Check sheet for the modelled part. Datum: model origin and axes. Units: mm. A direction names the side the tool comes from. Give positions to 0.01 mm unless a question says otherwise; leave off trailing zeros. Loops run counter-clockwise (first coordinate to the right, second up) from the corner with the lowest first, then second, coordinate; pieces in that order, holes last. Notation, with made-up numbers: (15, -5) - (61, -5) arc R29 ccw to (61, 19) - close; hole circle Ø4 at (-13.75, -36). An arc over 180 degrees is marked (long way). Answer in a Markdown table with one row per item. Add a question column.
(1) Sectioned sample at A-A on y = 3. Enter the section's corners in (x, z).
(2) Set-up check for faces 4 (the face through (0.29, 18.47, 10.58)), 5 (the face through (-3.779, -20, 1)), 6 (the face through (-22.382, 0, 7)): record each of +Z, -Z, +X, -X, +Y, -Y from which the full face is reachable in a straight line by a thin tool's end or side.
(3) Sectioned sample at C-C on z = -4.5. State how many separate pieces and enclosed holes the cut face has, then the cut area to 3 significant figures.
(4) Thickness scan on L1, parallel to X at y = 0, z = 11.1; L2, parallel to X at y = -15, z = 8.25; L3, parallel to Y at x = 5, z = -6. Record the ranges inside material, lowest first.
(5) Sectioned sample at B-B on x = -1. Enter the section's corners in (y, z).
(6) Sectioned sample at D-D on y = 12.5. Enter the section's corners in (x, z), then the cut area to 3 significant figures.
(7) Draft check along Z on faces 1 (the face through (-21.524, 0.071, 5.623)), 2 (the face through (18.721, -20, 1)), 3 (the face through (-4.344, -18.523, -2.422)). Enter one of: released by +Z, released by -Z, zero draft, split by the parting line, or undercut.
(8) Go/stop test with flat-tipped pins: P1, Ø0.5, axis at x = -8.5, y = -20.5, coming from the -Z side; P2, Ø3, axis at x = -15.5, y = -9, coming from the +Z side; P3, Ø12, axis at x = -13.5, z = 5, coming from the -Y side; P4, Ø3, axis at x = -11.5, z = -3.5, coming from the +Y side. Record where each tip stops, or that it passes through.
from build123d import *

# Parameters (mm, degrees)
PAD_DEPTH            = 20.6929
PAD001_DEPTH         = 1.692
PAD002_DEPTH         = 1.692
PAD003_START         = -1
SKETCH003_W          = 14.9418
SKETCH003_H          = 1.0711
PAD003_DEPTH         = 20.08
PAD004_DEPTH         = 1.1445
PAD005_DEPTH         = 1.1445
PAD006_DEPTH         = 1.1445
PAD007_DEPTH         = 1.1445
SKETCH008_R          = 18
SKETCH008_R_2        = 1.625
POCKET_DEPTH         = 21.0957
POCKET_DEPTH_BACK    = 0.4219
CHAMFER001_SIZE      = 0.7
SKETCH013_R          = 1.625
POCKET001_DEPTH      = 22.383
POCKET001_DEPTH_BACK = 22.383
BODY_PLACEMENT_ANGLE = 90


with BuildPart() as part:
    # Sketch → Pad (new body, symmetric)
    with BuildSketch(Plane.YZ):
        with BuildLine():
            ThreePointArc((0, 20.5122), (-0.4209, 0), (0, -20.5122))
            ThreePointArc((0, -20.5122), (0.44097, -21.514212), (1.445369, -21.949718))
            Line((1.445369, -21.949718), (11.0791, -22.292695))
            Line((11.0791, -22.292695), (11.0791, -20.791745))
            Line((1.498737, -20.450667), (11.0791, -20.791745))
            ThreePointArc((1.498737, 20.450667), (1.0791, 0), (1.498737, -20.450667))
            Line((1.498737, 20.450667), (11.0791, 20.791745))
            Line((11.0791, 20.791745), (11.0791, 22.292695))
            Line((1.445369, 21.949718), (11.0791, 22.292695))
            ThreePointArc((1.445369, 21.949718), (0.44097, 21.514212), (0, 20.5122))
        make_face()
    extrude(amount=PAD_DEPTH, both=True)

    # Sketch001 → Pad001 (join)
    with BuildSketch(Plane.YZ.offset(20.69)):
        with BuildLine():
            ThreePointArc((0, 20.5122), (-0.4209, 0), (0, -20.5122))
            ThreePointArc((0, -20.5122), (0.44097, -21.514212), (1.445369, -21.949718))
            Line((1.445369, -21.949718), (11.0791, -22.292695))
            Line((11.0791, 22.292695), (11.0791, -22.292695))
            Line((1.445369, 21.949718), (11.0791, 22.292695))
            ThreePointArc((1.445369, 21.949718), (0.44097, 21.514212), (0, 20.5122))
        make_face()
    extrude(amount=PAD001_DEPTH)

    # Sketch002 → Pad002 (join)
    with BuildSketch(Plane.YZ.offset(-20.69)):
        with BuildLine():
            ThreePointArc((0, 20.5122), (-0.4209, 0), (0, -20.5122))
            ThreePointArc((0, -20.5122), (0.44097, -21.514212), (1.445369, -21.949718))
            Line((1.445369, -21.949718), (11.0791, -22.292695))
            Line((11.0791, 22.292695), (11.0791, -22.292695))
            Line((1.445369, 21.949718), (11.0791, 22.292695))
            ThreePointArc((1.445369, 21.949718), (0.44097, 21.514212), (0, 20.5122))
        make_face()
    extrude(amount=-PAD002_DEPTH)

    # Sketch003 → Pad003 (join)
    with BuildSketch(Plane.XZ.offset(PAD003_START)):
        with Locations((-11.25, 20.36445)):
            Rectangle(SKETCH003_W, SKETCH003_H)
        with Locations((11.25, 20.36445)):
            Rectangle(SKETCH003_W, SKETCH003_H)
        with Locations((-11.25, -20.36445)):
            Rectangle(SKETCH003_W, SKETCH003_H)
        with Locations((11.25, -20.36445)):
            Rectangle(SKETCH003_W, SKETCH003_H)
    extrude(amount=-PAD003_DEPTH)

    # Sketch004 → Pad004 (join)
    with BuildSketch(Plane.YZ.offset(3.78)):
        Polygon((1.358658, 16.220017), (1.488, 19.8289), (21.0947, 19.8289), (21.0947, 19.7), align=None)
        Polygon((1.358658, -16.220017), (1.488, -19.8289), (21.0947, -19.8289), (21.0947, -19.7), align=None)
    extrude(amount=PAD004_DEPTH)

    # Sketch005 → Pad005 (join)
    with BuildSketch(Plane.YZ.offset(-3.78)):
        Polygon((1.358658, 16.220017), (1.488, 19.8289), (21.0947, 19.8289), (21.0947, 19.7), align=None)
        Polygon((1.358658, -16.220017), (1.488, -19.8289), (21.0947, -19.8289), (21.0947, -19.7), align=None)
    extrude(amount=-PAD005_DEPTH)

    # Sketch006 → Pad006 (join)
    with BuildSketch(Plane.YZ.offset(18.72)):
        Polygon((1.358658, 16.220017), (1.488, 19.8289), (21.0947, 19.8289), (21.0947, 19.7), align=None)
        Polygon((1.358658, -16.220017), (1.488, -19.8289), (21.0947, -19.8289), (21.0947, -19.7), align=None)
    extrude(amount=-PAD006_DEPTH)

    # Sketch007 → Pad007 (join)
    with BuildSketch(Plane.YZ.offset(-18.72)):
        Polygon((1.358658, 16.220017), (1.488, 19.8289), (21.0947, 19.8289), (21.0947, 19.7), align=None)
        Polygon((1.358658, -16.220017), (1.488, -19.8289), (21.0947, -19.8289), (21.0947, -19.7), align=None)
    extrude(amount=PAD007_DEPTH)

    # Sketch008 → Pocket (cut, two sides)
    with BuildSketch(Plane.XZ) as pocket_sk:
        Circle(SKETCH008_R)
        with Locations((15.750096, -15.750096)):
            Circle(SKETCH008_R_2)
    extrude(amount=-POCKET_DEPTH, mode=Mode.SUBTRACT)
    extrude(pocket_sk.sketch, amount=POCKET_DEPTH_BACK, mode=Mode.SUBTRACT)

    # Chamfer001
    chamfer001_edges = [part.edges().sort_by_distance(p)[0] for p in [
        (-20.69, 6.288919, 20.621206),
        (20.69, 6.288919, 20.621206),
        (21.53745, 11.0791, 22.292695),
        (-20.69, 6.288919, -20.621206),
    ]]
    chamfer(chamfer001_edges, length=CHAMFER001_SIZE)

    # Sketch013 → Pocket001 (cut, two sides)
    with BuildSketch(Plane.YZ) as pocket001_sk:
        with Locations((8, 0)):
            Circle(SKETCH013_R)
    extrude(amount=-POCKET001_DEPTH, mode=Mode.SUBTRACT)
    extrude(pocket001_sk.sketch, amount=POCKET001_DEPTH_BACK, mode=Mode.SUBTRACT)


with BuildPart() as part_1:
    # Body placement: moved
    add(part.part.moved(Location((0, 0, 12))).rotate(Axis((0, 0, 12), (-1, 0, 0)), BODY_PLACEMENT_ANGLE))


solid = part_1.part
Reply:
| question | item | result |
|---|---|---|
| 1 | outline | (-22.38, 0.92) - (-20.69, 0.92) - (-20.69, 10.91) - (-17.75, 10.91) - (-17.75, 12.41) - (-22.38, 12.41) - close; (17.75, 10.91) - (20.69, 10.91) - (20.69, 0.92) - (22.38, 0.92) - (22.38, 12.41) - (17.75, 12.41) - close |
| 2 | face 4 | none |
| 2 | face 5 | -Z |
| 2 | face 6 | +Z, -Z, -X, +Y, -Y |
| 3 | separate pieces | 4 |
| 3 | enclosed holes | 0 |
| 3 | area | 72.6 mm^2 |
| 4 | L1 | -22.38 to -18, 18 to 22.38 |
| 4 | L2 | -22.38 to -20.69, 20.69 to 22.38 |
| 4 | L3 | -20.9 to -19.83, 19.83 to 20.9 |
| 5 | outline | (-22.29, 0.92) - (-20.79, 0.92) - (-20.45, 10.5) arc R498.53 cw to (-17.97, 10.6) - (-17.97, 12.1) arc R500.03 ccw to (-20.51, 12) arc R1.5 ccw to (-21.95, 10.55) - close; (17.97, 10.6) arc R498.53 cw to (20.45, 10.5) - (20.79, 0.92) - (21.59, 0.92) - (22.27, 1.62) - (21.95, 10.55) arc R1.5 ccw to (20.51, 12) arc R500.03 ccw to (17.97, 12.1) - close |
| 6 | outline | (-22.38, 0.92) - (-20.69, 0.92) - (-20.69, 10.76) - (-12.95, 10.76) - (-12.95, 12.26) - (-22.38, 12.26) - close; (12.95, 10.76) - (20.69, 10.76) - (20.69, 0.92) - (22.38, 0.92) - (22.38, 12.26) - (12.95, 12.26) - close |
| 6 | area | 61.6 mm^2 |
| 7 | face 1 | undercut |
| 7 | face 2 | zero draft |
| 7 | face 3 | released by -Z |
| 8 | P1 | z = -9.08 |
| 8 | P2 | z = 12.36 |
| 8 | P3 | y = -22.29 |
| 8 | P4 | y = 20.9 |
